Autodesk Inventor part; units mm, degrees
ref_plane "YZ Plane" through (0, 0, 0) normal (1, 0, 0) x (0, 1, 0)
ref_plane "XZ Plane" through (0, 0, 0) normal (0, 1, 0) x (-1, 0, 0)
ref_plane "XY Plane" through (0, 0, 0) normal (0, 0, 1) x (1, 0, 0)
sketch "Sketch1" plane through (0, 0, 0) normal (0, 1, 0) x (-1, 0, 0)
  line L0 (9.5, -3) -> (-9.5, -3)
  line L1 (-9.5, -3) -> (-9.5, 3)
  line L2 (-9.5, 3) -> (9.5, 3)
  line L3 (9.5, 3) -> (9.5, -3)
  line L4 (9.5, -3) -> (-9.5, 3) construction
  line L5 (-9.5, -3) -> (9.5, 3) construction
  point P0 (0, 0)
  dimension "d0" = 19
  dimension "d1" = 6
extrude "Extrusion1" add sketch "Sketch1" along normal blind 6
sketch "Sketch2" plane through (-9.5, 0, 3) normal (0, 0, 1) x (1, 0, 0)
  line L0 (19, 6) -> (0, 6)
  arc A0 (4.5, 6) -> (14.5, 6) centre (9.5, 6) ccw
  point P0 (9.5, 0)
  point P1 (14.5, 6)
  dimension "d4" = 5
extrude "Extrusion2" add sketch "Sketch2" along normal blind 1 and the other way blind 7
sketch "Sketch3" plane through (-9.5, 0, 4) normal (0, 0, 1) x (1, 0, 0)
  line L0 (14.5, 6) -> (4.5, 6)
  point P0 (9.5, 0)
  point P1 (9.5, 6)
hole "Hole1" at (0, 6, 4) direction (0, 0, -1) diameter 7 end through all
sketch "Sketch4" plane through (0, 6, 0) normal (0, 1, 0) x (1, 0, 0)
  line L0 (-5, 3) -> (-9.5, 3)
  line L1 (9.5, 3) -> (5, 3)
  line L2 (-9.5, 3) -> (-9.5, -3)
  line L3 (9.5, -3) -> (9.5, 3)
  point P0 (0, 0)
  point P1 (-6, 0)
  point P2 (6, 0)
  dimension "d16" = 3
  dimension "d17" = 3
  dimension "d18" = 12
  dimension "d19" = 3.5
  dimension "d20" = 3.5
hole "Hole2" at (-6, 6, 0) at (6, 6, 0) direction (0, -1, 0) diameter 3 end through all
properties material "Brass, Soft Yellow, Welded"
CAD build for the part. Positions are in the model's coordinates, mm. A direction names the side the tool comes from. Round coordinates to 2 decimals unless told otherwise and drop trailing zeros. Order: outer loops, then holes, each group sorted by start corner. A loop starts at its lowest first (then second) coordinate and runs counter-clockwise, first axis right, second up. Notation, with made-up numbers: (32.5, 69.25) - (87.5, 69.25) arc R24 cw to (87.5, 94.25) - close; hole circle Ø11 at (52.25, -29.5). An arc over 180 degrees is marked (long way). Return JSON: item names as keys, results as strings.
(1) Cut at B-B (y = 0.5). Give the cut face in (x, z), then the cut area to 3 significant figures.
Answer key:
{"outline": "(-9.5, -3) - (9.5, -3) - (9.5, 3) - (-9.5, 3) - close; hole circle Ø3 at (-6, 0); hole circle Ø3 at (6, 0)", "area": "99.9 mm^2"}
(2) Pull direction X, two halves, no side cores. Call faces 4 (the face through (0.1, 1, 3.5)), 5 (the face through (0, 2, -4)), 6 (the face through (0.1, 2.5, -0.1)): +X half, -X half, draft (parallel to the pull), parting line (faces both ways), or undercut.
Answer key:
{"face 4": "parting line", "face 5": "draft", "face 6": "undercut"}
(3) Wall check: probe 1 along X at (y, z) = (1.8, 0); probe 2 along Z at (x, y) = (6, 1.45); probe 3 along X at (y, z) = (3.4, 0). Give the ranges that are in metal, low to high. Write a range as from..to.
Answer key:
{"probe 1": "x = -9.5..-7.5, -4.5..4.5, 7.5..9.5", "probe 2": "z = -3..-1.5, 1.5..3", "probe 3": "x = -9.5..-7.5, -4.5..-2.34, 2.34..4.5, 7.5..9.5"}
(4) Cut at C-C (z = -0.25). Give the cut face in (x, y), then the cut area to 3 significant figures.
Answer key:
{"outline": "(-9.5, 0) - (-7.48, 0) - (-7.48, 6) - (-9.5, 6) - close; (-4.52, 0) - (4.52, 0) - (4.52, 6) - (3.5, 6) arc R3.5 cw to (-3.5, 6) - (-4.52, 6) - close; (7.48, 0) - (9.5, 0) - (9.5, 6) - (7.48, 6) - close", "area": "59.3 mm^2"}
(5) Tool access for faces 1 (the face through (-9.5, 3, 0)), 2 (the face through (-0.1, 0.3, -3)), 3 (the face through (0.1, 0.3, 3)): list every direction of +Z, -Z, +X, -X, +Y, -Y with a clear straight run to the whole face (end or side of a thin tool).
Answer key:
{"face 1": "+Z, -Z, -X, +Y, -Y", "face 2": "-Z, -Y", "face 3": "+Z, -Y"}
(6) Cut at D-D (x = 0). Give the cut face in (y, z), then the cut area to 3 significant figures.
Answer key:
{"outline": "(0, -3) - (1, -3) - (1, -4) - (2.5, -4) - (2.5, 4) - (1, 4) - (1, 3) - (0, 3) - close", "area": "18.0 mm^2"}
(7) Pin check, flat tip, straight feed: pin 1 Ø2.5 at (x, z) = (-6, 0) entering from -Y. Stop position of the tip, or through.
Answer key:
{"pin 1": "passes through"}
(8) Cut at A-A (x = 6). Give the cut face in (y, z), then the cut area to 3 significant figures.
Answer key:
{"outline": "(0, -3) - (6, -3) - (6, -1.5) - (0, -1.5) - close; (0, 1.5) - (6, 1.5) - (6, 3) - (0, 3) - close", "area": "18.0 mm^2"}
